from build123d import *

# Parameters (mm, degrees)
BOSS_EXTRUDE1_DEPTH     = 2.54
F_8_CLEARANCE_HOLE1_D   = 4.4958
F_1_4_CLEARANCE_HOLE1_D = 6.7564
SKETCH6_R               = 10.16
CUT_EXTRUDE1_DEPTH      = 163.659188489


with BuildPart() as part:
    # Sketch1 → Boss-Extrude1 (new body)
    with BuildSketch(Plane(origin=(0, 0, 0), x_dir=(1, 0, 0), z_dir=(0, 1, 0))):
        with BuildLine():
            Line((26.3525, 125.73), (100.965, 26.246666667))
            ThreePointArc((100.965, 26.246666667), (101.437069471, 25.345689824), (101.6, 24.341666667))
            Line((101.6, 24.341666667), (101.6, 3.175))
            ThreePointArc((101.6, 3.175), (100.67006403, 0.92993597), (98.425, 0))
            Line((98.425, 0), (23.8125, 0))
            ThreePointArc((23.8125, 0), (21.56743597, 0.92993597), (20.6375, 3.175))
            Line((20.6375, 3.175), (20.6375, 73.025))
            ThreePointArc((20.6375, 73.025), (19.70756403, 75.27006403), (17.4625, 76.2))
            Line((17.4625, 76.2), (3.175, 76.2))
            ThreePointArc((3.175, 76.2), (0.92993597, 77.12993597), (0, 79.375))
            Line((0, 79.375), (0, 123.825))
            ThreePointArc((0, 123.825), (0.92993597, 126.07006403), (3.175, 127))
            Line((3.175, 127), (23.8125, 127))
            ThreePointArc((23.8125, 127), (25.232403166, 126.664806331), (26.3525, 125.73))
        make_face()
    extrude(amount=BOSS_EXTRUDE1_DEPTH)

    # #8 Clearance Hole1 (through all)
    with Locations(Plane.XZ):
        with Locations((38.1, -12.7), (63.5, -12.7), (88.9, -12.7), (12.7, -88.9), (12.7, -114.3)):
            Hole(F_8_CLEARANCE_HOLE1_D / 2)

    # 1/4 Clearance Hole1 (through all)
    with Locations(Plane.XZ):
        with Locations((30.9, -64.9), (30.9, -30.9), (64.9, -30.9), (64.9, -64.9)):
            Hole(F_1_4_CLEARANCE_HOLE1_D / 2)

    # Sketch6 → Cut-Extrude1 (cut, through all)
    with BuildSketch(Plane.XZ):
        with Locations(Location((47.9, -47.9, 0), (0, 0, 270))):
            Circle(SKETCH6_R)
        with BuildLine():
            Line((76.0125, -22.225), (88.9, -22.225))
            ThreePointArc((88.9, -22.225), (90.319903166, -23.102548417), (90.17, -24.765))
            Line((90.17, -24.765), (77.2825, -41.948333333))
            ThreePointArc((77.2825, -41.948333333), (75.510488421, -42.501868069), (74.425, -40.995833333))
            Line((74.425, -40.995833333), (74.425, -23.8125))
            ThreePointArc((74.425, -23.8125), (74.889967985, -22.689967985), (76.0125, -22.225))
        make_face()
        with BuildLine():
            Line((30.7975, -103.928333333), (49.115, -79.505))
            ThreePointArc((49.115, -79.505), (49.414806331, -76.180096834), (46.575, -74.425))
            Line((46.575, -74.425), (41.275, -74.425))
            ThreePointArc((41.275, -74.425), (27.804615818, -80.004615818), (22.225, -93.475))
            Line((22.225, -93.475), (22.225, -101.070833333))
            ThreePointArc((22.225, -101.070833333), (25.481465264, -105.58893754), (30.7975, -103.928333333))
        make_face()
    extrude(amount=-CUT_EXTRUDE1_DEPTH, mode=Mode.SUBTRACT)


solid = part.part
Model file for the job. Use its own axes, mm. A direction names the side the tool comes from. Give positions to 0.01 mm unless a question says otherwise; leave off trailing zeros. Order: outer loops, then holes, each group sorted by start corner. A loop starts at its lowest first (then second) coordinate and runs counter-clockwise, first axis right, second up. Notation, with made-up numbers: (29, 38.25) - (81, 38.25) arc R17 cw to (81, 65.25) - close; hole circle Ø9 at (-33.75, -19.75). An arc over 180 degrees is marked (long way). Write item = value, one per line. Start each with the question number.
1. Two-plate mould, pull along X, no slides. Class faces 3 (the flat face through (10, 1, -76.2)), 4 (the cylindrical face through (0.95, 1.25, -77.11)), 5 (the cylindrical face through (36.024, 1.288, -13.561)), 6 (the cylindrical face through (25.214, 1.252, -126.674)): pulls with the +X half, pulls with the -X half, needs draft (parallel to the pull), parting line crosses it, or undercut.
2. Cut at C-C, the plane y = 1.6. State how many separate pieces and enclosed holes the cut face has, and give its area (3 significant figures).
3. Cut at B-B, the plane z = -47.9. List the corners of the cut face in (x, y) (1 decimal), and give its area (3 significant figures).
4. Drop flat-ended pins along their axis: P1, Ø1, axis at x = 48, y = 1, coming from the -Z side; P2, Ø0.8, axis at x = 85, y = 1, coming from the -Z side. Give the stop position or say it passes through.
5. Which spindle directions (+Z, -Z, +X, -X, +Y, -Y) get a long thin tool onto all of the face, cutting with end or side? Do faces 1 (the flat face through (44, 1, -74.425)), 2 (the flat face through (52, 0, -64)). Say none if no direction does.
6. Cut at D-D, the plane z = -70. List the corners of the cut face in (x, y), and give its area (3 significant figures).
7. Probe line 1 along X through (y, z) = (1.4, -13); line 2 along Z through (x, y) = (64, 2.45); line 3 along Z through (x, y) = (48, 2). List the from-to ranges inside material, lowest first.
8. Cut at A-A, the plane z = -88.9. List the corners of the cut face in (x, y) (3 decimals).
Taken from the geometry:
q1.face_3 = needs draft
q1.face_4 = pulls with the -X half
q1.face_5 = undercut
q1.face_6 = pulls with the +X half
q2.separate_pieces = 1
q2.enclosed_holes = 12
q2.area = 6,200 mm²
q3.outline = (20.6, 0) - (37.7, 0) - (37.7, 2.5) - (20.6, 2.5) - close; (58.1, 0) - (84.7, 0) - (84.7, 2.5) - (58.1, 2.5) - close
q3.area = 111 mm²
q4.P1 = -97.53
q4.P2 = -48.07
q5.face_1 = +Y, -Y
q5.face_2 = +Z, -Z, +X, -X, -Y
q6.outline = (20.64, 0) - (68.15, 0) - (68.15, 2.54) - (20.64, 2.54) - close
q6.area = 121 mm²
q7.line_1 = 20.64 to 35.87, 40.33 to 61.27, 65.73 to 86.67, 91.13 to 101.6
q7.line_2 = -75.53 to -68.16, -61.64 to -34.16, -27.64 to -14.89, -10.51 to 0
q7.line_3 = -96.87 to -80.99, -74.76 to -58.06, -37.74 to 0
q8.outline = (0, 0) - (10.452, 0) - (10.452, 2.54) - (0, 2.54) - close; (14.948, 0) - (22.783, 0) - (22.783, 2.54) - (14.948, 2.54) - close; (42.069, 0) - (53.975, 0) - (53.975, 2.54) - (42.069, 2.54) - close
